Print and shaded views of the part. All mm, measured from the part's lowest x, y and z. Round coordinates to 2 decimals unless told otherwise and drop trailing zeros. Loops run counter-clockwise (first coordinate to the right, second up) from the corner with the lowest first, then second, coordinate; pieces in that order, holes last. Notation, with made-up numbers: (10, 21) - (34, 21) arc R12 cw to (34, 38) - close; hole circle Ø4 at (61, 24.25). An arc over 180 degrees is marked (long way). Use one line per item in the form item = value.
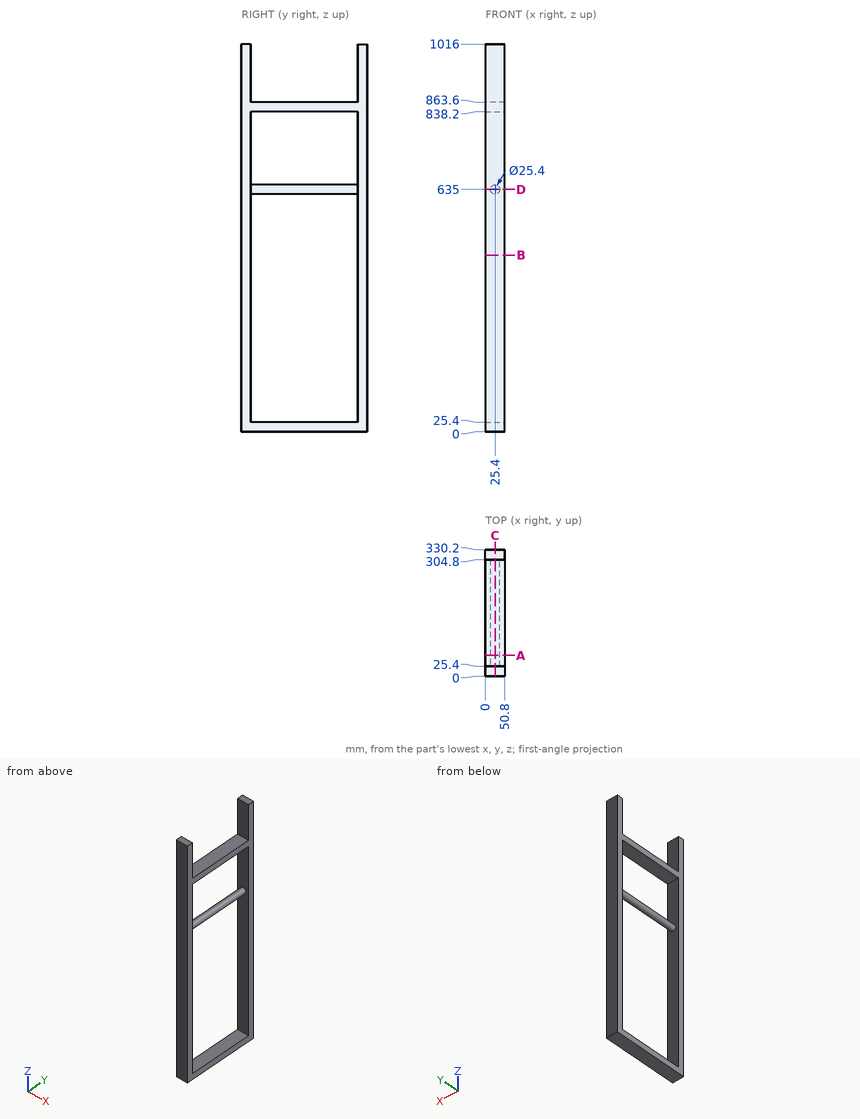
1) Slice it at B-B (z = 463). Write the cut outline in (x, y), plus the area to 3 significant figures.
Report:
outline = (0, 0) - (50.8, 0) - (50.8, 25.4) - (0, 25.4) - close; (0, 304.8) - (50.8, 304.8) - (50.8, 330.2) - (0, 330.2) - close
area = 2,580 mm^2
2) Flat gauge pins, fed straight in: pin 1 (6 mm diameter, centred on x = 26, y = 252, fed in from +Z); pin 2 (1.5 mm diameter, centred on y = 125, z = 642.5, fed in from +X). Where does each tip first touch, or does it go through?
Report:
pin_1 = 863.6
pin_2 = 36.16
3) Slice it at C-C (x = 25.4). Write the cut outline in (y, z), plus the area to 3 significant figures.
Report:
outline = (0, 0) - (330.2, 0) - (330.2, 1016) - (304.8, 1016) - (304.8, 863.6) - (25.4, 863.6) - (25.4, 1016) - (0, 1016) - close; hole (25.4, 25.4) - (304.8, 25.4) - (304.8, 622.3) - (25.4, 622.3) - close; hole (25.4, 647.7) - (304.8, 647.7) - (304.8, 838.2) - (25.4, 838.2) - close
area = 72,900 mm^2
4) Slice it at A-A (y = 54). Write the cut outline in (x, z).
Report:
outline = (0, 0) - (50.8, 0) - (50.8, 25.4) - (0, 25.4) - close; (0, 838.2) - (50.8, 838.2) - (50.8, 863.6) - (0, 863.6) - close; circle Ø25.4 at (25.4, 635)
5) Slice it at D-D (z = 635). Write the cut outline in (x, y).
Report:
outline = (0, 0) - (50.8, 0) - (50.8, 25.4) - (38.1, 25.4) - (38.1, 304.8) - (50.8, 304.8) - (50.8, 330.2) - (0, 330.2) - (0, 304.8) - (12.7, 304.8) - (12.7, 25.4) - (0, 25.4) - close
6) Drill centre lines: probe 1 along Y at (x, z) = (13, 395); probe 2 along Z at (x, y) = (48.5, 39.5); probe 3 along Z at (x, y) = (30, 297). Where is each one in solid material? Low to high.
Report:
probe_1 = 0 to 25.4, 304.8 to 330.2
probe_2 = 0 to 25.4, 838.2 to 863.6
probe_3 = 0 to 25.4, 623.16 to 646.84, 838.2 to 863.6
